For this review, use the dimensioned drawing (mm, ordinates from the lowest corner) and the shaded views. A direction names the side the tool comes from. Round coordinates to 2 decimals unless told otherwise and drop trailing zeros. Loops run counter-clockwise (first coordinate to the right, second up) from the corner with the lowest first, then second, coordinate; pieces in that order, holes last. Notation, with made-up numbers: (-16, 9) -> (33, 9) arc R19 ccw to (33, 13) -> close; hole circle Ø4 at (-36, -39). An arc over 180 degrees is marked (long way). Answer as CSV lines item,"result". Start each with the question number.
(1) Take a section at C-C, the plane z = 64. Write out the cut boundary in (x, y), and give its area (3 significant figures).
(2) To check wall thickness, follow line 1 (Z direction, x = 77.5, y = 20.5); line 2 (Z direction, x = 33, y = 24.5); line 3 (X direction, y = 58, z = 106.5). State the ranges of each line that lie inside material, in increasing order. Write a range as from..to.
(3) Machinability: for the marked faces 1 and 2, which of the approach directions +Z, -Z, +X, -X, +Y, -Y give a long, thin tool a straight path to every point of the face, cutting with its end or side? Answer none if there is none.
(4) Take a section at A-A, the plane x = 26. Write out the cut boundary in (y, z), and give its area (3 significant figures).
(5) Take a section at B-B, the plane y = 18. Write out the cut boundary in (x, z).
(6) Take a section at D-D, the plane y = 50. Write out the cut boundary in (x, z).
(7) For P1, Ø1.5, axis at x = 44.5, z = 117, coming from the -Y side; P2, Ø8, axis at x = 50, y = 32, coming from the -Z side; P3, Ø4, axis at x = 40.5, z = 123.5, coming from the -Y side; P4, Ø6, axis at x = 30, y = 87, coming from the +Z side, all flat-tipped, find the tip position at first contact; note any pin that passes through.
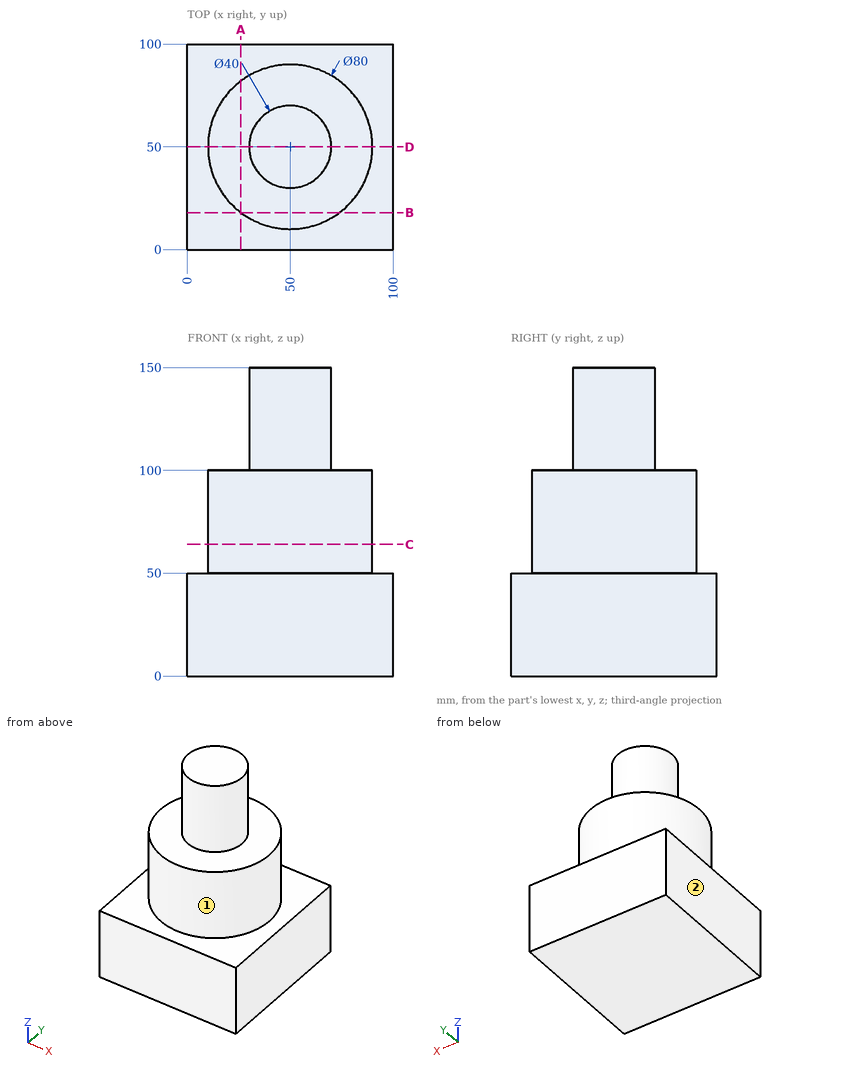
The answers:
1,outline,"circle Ø80 at (50, 50)"
1,area,"5,030 mm²"
2,line 1,"0..50"
2,line 2,"0..100"
2,line 3,"31.67..68.33"
3,face 1,"+Z"
3,face 2,"+Z, -Z, -X, +Y, -Y"
4,outline,"(0, 0) -> (100, 0) -> (100, 50) -> (82, 50) -> (82, 100) -> (18, 100) -> (18, 50) -> (0, 50) -> close"
4,area,"8,200 mm²"
5,outline,"(0, 0) -> (100, 0) -> (100, 50) -> (74, 50) -> (74, 100) -> (26, 100) -> (26, 50) -> (0, 50) -> close"
6,outline,"(0, 0) -> (100, 0) -> (100, 50) -> (90, 50) -> (90, 100) -> (70, 100) -> (70, 150) -> (30, 150) -> (30, 100) -> (10, 100) -> (10, 50) -> (0, 50) -> close"
7,P1,"y = 30.57"
7,P2,"z = 0"
7,P3,"y = 31.46"
7,P4,"z = 100"
